Here's how the part is built. I have some questions about the finished solid (model axes, mm). A direction names the side the tool comes from. Round coordinates to 2 decimals unless told otherwise and drop trailing zeros. Write each loop counter-clockwise with the first axis right and the second up, starting at its lowest first coordinate (ties: lowest second). Pieces come first, ordered by that corner, then holes. Notation, with made-up numbers: (47, 49) -> (68, 49) arc R8 ccw to (68, 62) -> close; hole circle Ø11 at (-1, 67). An arc over 180 degrees is marked (long way). Put each result on its own line as item: value. Start each with the question number.
1) If I drill on line 1 along X through (y, z) = (6, 2) (3 decimals); line 2 along Y through (x, z) = (8.5, 2.5); line 3 along Y through (x, z) = (74.5, 0), over which ranges is the centre line in solid material (lowest first)? Write a range as [from, to].
2) I want a section at A-A, the plane y = 0. List the corners of the cut face in (x, z) for me.
3) We'd pull the mould along Y, two halves only. Please class faces 4 (the flat face through (10.73, 0.1, 0.04)), 5 (the flat face through (49.3, 10.05, 1.52)), 6 (the conical face through (-8.668, -3.314, -2.854)), 7 (the flat face through (37, 6, -3)): released by +Y, released by -Y, zero draft, split by the parting line, or undercut.
4) Which directions (+Z, -Z, +X, -X, +Y, -Y) give clear straight access to the entire face, cutting with the end or side of a thin tool? Please do faces 1 (the flat face through (6.194, -0.704, -1.521)), 2 (the flat face through (6.177, -0.687, 1.479)), 3 (the flat face through (49.3, 10.074, -1.479)).
5) I want a section at C-C, the plane x = 63.5. List the corners of the cut face in (y, z) for me, then the cut area to 3 significant figures.
6) I want a section at B-B, the plane z = -1.5. List the corners of the cut face in (x, y) for me, then the cut area to 3 significant figures.
7) Will this pin go through, and if not, where does the flat tip stop? P1, Ø2, axis at x = 16.5, y = 1.5, coming from the +Z side.
from build123d import *


with BuildPart() as part:
    # Base-Sweep: sweep along a path in Sketch1
    with BuildLine(Plane.XY) as base_sweep_path:
        Line((100, 4), (0, 4))
        ThreePointArc((0, 4), (-3.69551813, -1.530733729), (2.828427125, -2.828427125))
        Line((2.828427125, -2.828427125), (8.242640687, 2.585786438))
    # Sketch2 → Base-Sweep (sweep)
    with BuildSketch(Plane(origin=(100, 4, 0), x_dir=(0, 0, 1), z_dir=(-1, 0, 0))):
        Polygon((-3, 5.196152423), (0, 6.92820323), (3, 5.196152423), (3, 1.732050808), (0, 0), (-3, 1.732050808), align=None)
    sweep(path=base_sweep_path.line)


solid = part.part
Findings:
1. line 1: x = [-7.715, 100]
1. line 2: y = [-4.91, 0.8], [5.44, 9.48]
1. line 3: y = [4, 10.93]
2. outline: (-10.93, 0) -> (-9.2, -3) -> (-5.73, -3) -> (-4, 0) -> (-5.73, 3) -> (-9.2, 3) -> close; (5.66, 0) -> (8.11, -3) -> (10.83, -3) -> (10.83, 3) -> (8.11, 3) -> close
3. face 4: undercut
3. face 5: released by +Y
3. face 6: split by the parting line
3. face 7: zero draft
4. face 1: -Z
4. face 2: +Z
4. face 3: -Z, +X, -X, +Y
5. outline: (4, 0) -> (5.73, -3) -> (9.2, -3) -> (10.93, 0) -> (9.2, 3) -> (5.73, 3) -> close
5. area: 31.2 mm2
6. outline: (0, 4.87) -> (100, 4.87) -> (100, 10.06) -> (0, 10.06) arc R10.06 ccw (long way) to (7.12, -7.12) -> (12.53, -1.7) -> (8.86, 1.97) -> (3.44, -3.44) arc R4.87 cw (long way) to start
6. area: 712 mm2
7. P1: passes through
